from build123d import *

# Parameters (mm, degrees)
SKETCH_1_W          = 7
SKETCH_1_H          = 15
EXTRUDE_1_DEPTH     = 10
SKETCH_2_R          = 2
CUT_EXTRUDE_1_DEPTH = 16
SKETCH_3_R          = 0.5
CUT_EXTRUDE_2_DEPTH = 8


with BuildPart() as part:
    # 草图1 → 凸台-拉伸1 (new body)
    with BuildSketch(Plane(origin=(0, 0, 0), x_dir=(1, 0, 0), z_dir=(0, 1, 0))):
        with Locations((3.5, 7.5)):
            Rectangle(SKETCH_1_W, SKETCH_1_H)
    extrude(amount=EXTRUDE_1_DEPTH)

    # 草图2 → 切除-拉伸1 (cut, through all)
    with BuildSketch(Plane.XY):
        with Locations((4, 4)):
            Circle(SKETCH_2_R)
    extrude(amount=-CUT_EXTRUDE_1_DEPTH, mode=Mode.SUBTRACT)

    # 草图3 → 切除-拉伸2 (cut)
    with BuildSketch(Plane(origin=(0, 10, 0), x_dir=(1, 0, 0), z_dir=(0, 1, 0))):
        with Locations((1, 7.5)):
            Circle(SKETCH_3_R)
    extrude(amount=-CUT_EXTRUDE_2_DEPTH, mode=Mode.SUBTRACT)


solid = part.part
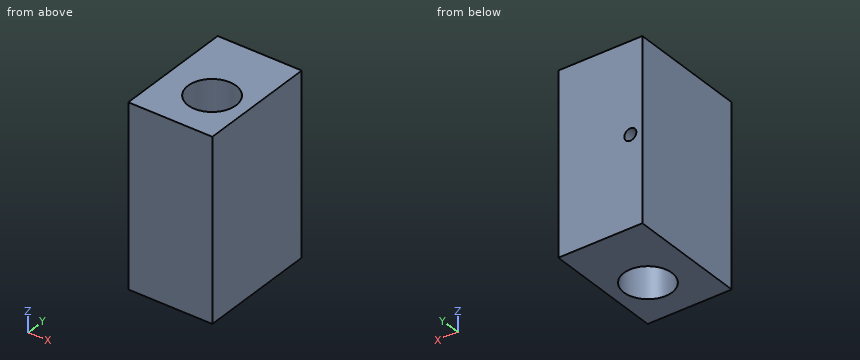
Could you check a few things on this model? Use its own coordinates, in mm. Give positions to 0.01 mm unless a question says otherwise; leave off trailing zeros. Write each loop counter-clockwise with the first axis right and the second up, starting at its lowest first coordinate (ties: lowest second). Pieces come first, ordered by that corner, then holes. Notation, with made-up numbers: (13, -7.75) -> (37, -7.75) arc R17 ccw to (37, 17.25) -> close; hole circle Ø9 at (-11.5, 36). An arc over 180 degrees is marked (long way). Answer as CSV lines item,"result". Start each with the question number.
(1) If we section it at A-A, the plane y = 4: Write out the boundary of the cut face in (x, z).
(2) If we section it at B-B, the plane x = 4: Write out the boundary of the cut face in (y, z).
(3) If we section it at C-C, the plane z = -8.75: Write out the boundary of the cut face in (x, y), and give its area (3 significant figures).
(4) If we section it at D-D, the plane x = 1: Write out the boundary of the cut face in (y, z), and give its area (3 significant figures).
(5) Please list where these lines run through material, in increasing order: line 1 (Z direction, x = 1, y = 6.25); line 2 (X direction, y = 5.75, z = -7.5); line 3 (Y direction, x = 4, z = -8.75).
Answer list:
1,outline,"(0, -15) -> (2, -15) -> (2, 0) -> (0, 0) -> close; (6, -15) -> (7, -15) -> (7, 0) -> (6, 0) -> close; hole circle Ø1 at (1, -7.5)"
2,outline,"(0, -15) -> (2, -15) -> (2, 0) -> (0, 0) -> close; (6, -15) -> (10, -15) -> (10, 0) -> (6, 0) -> close"
3,outline,"(0, 0) -> (7, 0) -> (7, 10) -> (0, 10) -> close; hole circle Ø4 at (4, 4)"
3,area,"57.4 mm^2"
4,outline,"(0, -15) -> (10, -15) -> (10, -8) -> (2, -8) -> (2, -7) -> (10, -7) -> (10, 0) -> (0, 0) -> close"
4,area,"142 mm^2"
5,line 1,"-15 to -8, -7 to 0"
5,line 2,"0 to 0.5, 1.5 to 3.03, 4.97 to 7"
5,line 3,"0 to 2, 6 to 10"
